Read the model definition and answer for the solid it produces. Units are mm, in the model's axes. A direction names the side the tool comes from. Coordinates: 2 decimals unless noted, no trailing zeros. Write each loop counter-clockwise with the first axis right and the second up, starting at its lowest first coordinate (ties: lowest second). Pieces come first, ordered by that corner, then holes.
1) Find the intervals of material crossed by line 1 (X direction, y = 1, z = 1.75); line 2 (Y direction, x = 65.5, z = 9); line 3 (Z direction, x = 25, y = -5), in increasing order.
2) The part is cut by section B-B (y = -20). Determine the outline of the cut face in (x, z), then the cut area to 3 significant figures.
3) Which of the six approach directions +Z, -Z, +X, -X, +Y, -Y give full straight-line access (tool end or side, diameter ignored) to faces 4 (the face through (-2, 3.25, 8)), 5 (the face through (-1.7, 5, 18.5)), 6 (the face through (-1.62, -9.16, 6.09))?
4) Each of these flat-tipped pins is pushed along its axis until it touches: pin 1 Ø1.2 at (x, z) = (-38.5, 22) entering from -Y; pin 2 Ø4 at (x, z) = (32, 20) entering from +Y; pin 3 Ø3.5 at (x, z) = (13, 10.5) entering from +Y. Where does it stop, or does it pass through?
5) The part is cut by section A-A (x = -81.5). Determine the outline of the cut face in (y, z), then the cut area to 3 significant figures.
6) The part is cut by section C-C (y = 24). Determine the outline of the cut face in (x, z), then the cut area to 3 significant figures.
7) Determine the mould class of faces 1 (the face through (-1.62, 9.16, 6.09)), 2 (the face through (-2, 0, 25.5)), 3 (the face through (-119.4, 0, 13)) for opening direction Z: +Z half, -Z half, draft (parallel to the pull), parting line (faces both ways), or undercut.
from build123d import *

# Parameters (mm, degrees)
BOSS_EXTRUDE1_DEPTH      = 119.4
BOSS_EXTRUDE1_DEPTH_BACK = 119.4
SKETCH1_W                = 230.8
SKETCH1_H                = 6.5
CUT_EXTRUDE1_DEPTH       = 20
SHELL1_START             = -115.4
SHELL1_DEPTH             = 230.8
CHAMFER1_SIZE            = 4


# Read off the part's stored shape, not the designer's step: Shell1
with BuildPart() as part:
    # Sketch4 → Boss-Extrude1 (new, two sides: drawn at the far end of the back side and taken through both)
    with BuildSketch(Plane(origin=(0, 0, 0), x_dir=(0, 0, -1), z_dir=(1, 0, 0)).offset(-BOSS_EXTRUDE1_DEPTH_BACK)):
        Polygon((0, 7.25), (-25.5, 30), (-25.5, -30), (0, -7.25), align=None)
        Polygon((-23.5, 6), (-23.5, -6), (-19.5, -6), (-13.5, 0), (-19.5, 6), align=None, mode=Mode.SUBTRACT)
    extrude(amount=BOSS_EXTRUDE1_DEPTH + BOSS_EXTRUDE1_DEPTH_BACK)

    # Sketch1 → Cut-Extrude1 (cut)
    with BuildSketch(Plane.XY):
        Rectangle(SKETCH1_W, SKETCH1_H)
    extrude(amount=CUT_EXTRUDE1_DEPTH, mode=Mode.SUBTRACT)

    # Shell1 outline → Shell1 (cut)
    with BuildSketch(Plane.YZ.offset(SHELL1_START)):
        Polygon((-10, 21.5), (-26.431372549, 21.5), (-10.818627451, 4), (-7.25, 4), (-7.25, 15.093145751), (-10, 17.843145751), align=None)
        Polygon((26.431372549, 21.5), (10, 21.5), (10, 17.843145751), (7.25, 15.093145751), (7.25, 4), (10.818627451, 4), align=None)
    extrude(amount=SHELL1_DEPTH, mode=Mode.SUBTRACT)

    # Chamfer1
    # the kernel refuses this chamfer: 4 mm, written as the material it adds along each edge
    with BuildSketch(Plane(origin=(-115.4, -7.25, 4), x_dir=(0, -0.9996219169112968, -0.02749587661058638), z_dir=(1, 0, 0))) as chamfer1_piece_1_section:
        Polygon((CHAMFER1_SIZE * 0.999621916911, -CHAMFER1_SIZE * 0.0274958766106), (-CHAMFER1_SIZE * 0.0274958766106, -CHAMFER1_SIZE * 0.999621916911), (0, 0), align=None)
    chamfer1_piece_1 = extrude(amount=230.8, mode=Mode.PRIVATE)
    chamfer1_piece_1 = split(chamfer1_piece_1, bisect_by=Plane(origin=(0, -10.469830587, 3.609040878), z_dir=(0, 0.7461972096049123, 0.6657249615102642)), keep=Keep.TOP, mode=Mode.PRIVATE)
    add(chamfer1_piece_1)
    with BuildSketch(Plane(origin=(-115.4, 7.25, 4), x_dir=(0, 0.9996219169112968, -0.02749587661058638), z_dir=(1, 0, 0))) as chamfer1_piece_2_section:
        Polygon((CHAMFER1_SIZE * 0.999621916911, CHAMFER1_SIZE * 0.0274958766106), (-CHAMFER1_SIZE * 0.0274958766106, CHAMFER1_SIZE * 0.999621916911), (0, 0), align=None)
    chamfer1_piece_2 = extrude(amount=230.8, mode=Mode.PRIVATE)
    chamfer1_piece_2 = split(chamfer1_piece_2, bisect_by=Plane(origin=(0, 10.469830587, 3.609040878), z_dir=(0, -0.7461972096049116, 0.6657249615102648)), keep=Keep.TOP, mode=Mode.PRIVATE)
    add(chamfer1_piece_2)


solid = part.part
Reported:
1. line 1: x = -119.4 to -115.4, 115.4 to 119.4
1. line 2: y = -7.25 to -3.25, 3.25 to 7.25
1. line 3: z = 0 to 18.5, 23.5 to 25.5
2. outline: (-119.4, 14.29) - (-115.4, 14.29) - (-115.4, 21.5) - (115.4, 21.5) - (115.4, 14.29) - (119.4, 14.29) - (119.4, 25.5) - (-119.4, 25.5) - close
2. area: 1,010 mm2
3. face 4: -Z
3. face 5: +X, -X
3. face 6: -Y
4. pin 1: stops at y = -27.41
4. pin 2: stops at y = 26.88
4. pin 3: stops at y = 7.25
5. outline: (-30, 25.5) - (-26.43, 21.5) - (-10, 21.5) - (-10, 17.84) - (-7.25, 15.09) - (-7.25, 8) - (-11.02, 4.23) - (-7.25, 0) - (-3.25, 0) - (-3.25, 16.75) - (-6, 19.5) - (-6, 23.5) - (6, 23.5) - (6, 19.5) - (3.25, 16.75) - (3.25, 0) - (7.25, 0) - (11.02, 4.23) - (7.25, 8) - (7.25, 15.09) - (10, 17.84) - (10, 21.5) - (26.43, 21.5) - (30, 25.5) - close
5. area: 413 mm2
6. outline: (-119.4, 18.77) - (-115.4, 18.77) - (-115.4, 21.5) - (115.4, 21.5) - (115.4, 18.77) - (119.4, 18.77) - (119.4, 25.5) - (-119.4, 25.5) - close
6. area: 977 mm2
7. face 1: undercut
7. face 2: +Z half
7. face 3: draft
